```python
from build123d import *

# Parameters (mm, degrees)
SKETCH_R        = 4.3
SKETCH_R_2      = 2.8
PAD_DEPTH       = 10
SKETCH001_R     = 4.5
POCKET_DEPTH    = 5
FILLET_R        = 4
SKETCH002_R     = 4.3
POCKET001_DEPTH = 10.001


with BuildPart() as part:
    # Sketch → Pad (new body)
    with BuildSketch(Plane.XY):
        Polygon((0.4, 0), (177.6, 0), (177.6, 70), (115.6, 70), (115.6, 96.6), (-19, 96.6), (-19, 70.4), (0.4, 70.4), align=None)
        with Locations((15, 60)):
            Circle(SKETCH_R, mode=Mode.SUBTRACT)
        with Locations((15, 10)):
            Circle(SKETCH_R, mode=Mode.SUBTRACT)
        with Locations((170, 47)):
            Circle(SKETCH_R_2, mode=Mode.SUBTRACT)
        with Locations((170, 23)):
            Circle(SKETCH_R_2, mode=Mode.SUBTRACT)
    extrude(amount=PAD_DEPTH)

    # Sketch001 (on Face14 of Pad) → Pocket (cut)
    with BuildSketch(Plane.XY.offset(10)):
        with Locations((170, 47)):
            Circle(SKETCH001_R)
        with Locations((170, 23)):
            Circle(SKETCH001_R)
    extrude(amount=-POCKET_DEPTH, mode=Mode.SUBTRACT)

    # Fillet
    fillet_edges = [part.edges().sort_by_distance(p)[0] for p in [
        (115.6, 70, 5),
    ]]
    fillet(fillet_edges, radius=FILLET_R)

    # Sketch002 (on Face15 of Fillet) → Pocket001 (cut, through all)
    with BuildSketch(Plane.XY.offset(10)):
        with Locations((-11.5, 84.1)):
            Circle(SKETCH002_R)
        with Locations((23.5, 84.1)):
            Circle(SKETCH002_R)
        with Locations((103.1, 84.1)):
            Circle(SKETCH002_R)
    extrude(amount=-POCKET001_DEPTH, mode=Mode.SUBTRACT)


solid = part.part
```
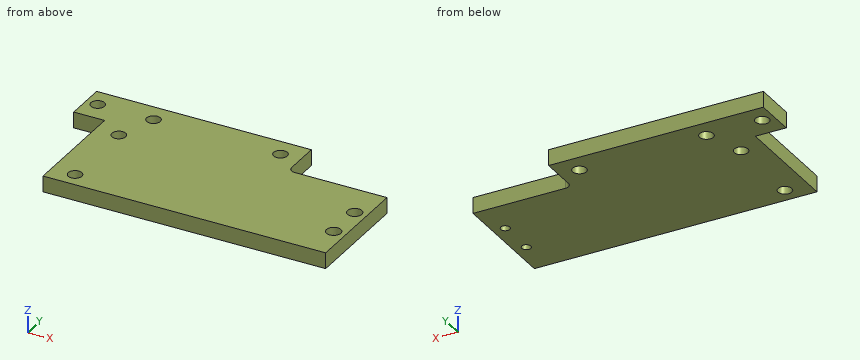
CAD build for the part. Positions are in the model's coordinates, mm. Give positions to 0.01 mm unless a question says otherwise; leave off trailing zeros. Loops run counter-clockwise (first coordinate to the right, second up) from the corner with the lowest first, then second, coordinate; pieces in that order, holes last. Notation, with made-up numbers: (-1, 57.5) - (4, 57.5) arc R19 cw to (4, 92.5) - close; hole circle Ø1 at (-29, 12.5). An arc over 180 degrees is marked (long way). Put each result on its own line as item: value.
Q1. Flat gauge pins, fed straight in: pin 1 (7 mm diameter, centred on x = 170, y = 23, fed in from +Z); pin 2 (5 mm diameter, centred on x = -8.5, z = 6.5, fed in from -Y); pin 3 (5 mm diameter, centred on y = 84, z = 5.5, fed in from +X); pin 4 (5 mm diameter, centred on x = 23.5, y = 84.1, fed in from -Z). Where does each tip first touch, or does it go through?
Filled in:
pin 1: stops at z = 5
pin 2: stops at y = 70.4
pin 3: stops at x = 115.6
pin 4: passes through
Q2. Slice it at B-B (y = 60). Give the cut face in (x, z), plus the area to 3 significant figures.
Filled in:
outline: (0.4, 0) - (10.7, 0) - (10.7, 10) - (0.4, 10) - close; (19.3, 0) - (177.6, 0) - (177.6, 10) - (19.3, 10) - close
area: 1,690 mm²
Q3. Slice it at A-A (y = 84.1). Give the cut face in (x, z).
Filled in:
outline: (-19, 0) - (-15.8, 0) - (-15.8, 10) - (-19, 10) - close; (-7.2, 0) - (19.2, 0) - (19.2, 10) - (-7.2, 10) - close; (27.8, 0) - (98.8, 0) - (98.8, 10) - (27.8, 10) - close; (107.4, 0) - (115.6, 0) - (115.6, 10) - (107.4, 10) - close
Q4. Probe line 1 along Y through (x, z) = (170, 3.45); line 2 along Y through (x, z) = (15, 2); line 3 along Y through (x, z) = (-11.5, 6). List the from-to ranges inside material, lowest first.
Filled in:
line 1: y = 0 to 20.2, 25.8 to 44.2, 49.8 to 70
line 2: y = 0 to 5.7, 14.3 to 55.7, 64.3 to 96.6
line 3: y = 70.4 to 79.8, 88.4 to 96.6
Q5. Slice it at C-C (x = 15). Give the cut face in (y, z).
Filled in:
outline: (0, 0) - (5.7, 0) - (5.7, 10) - (0, 10) - close; (14.3, 0) - (55.7, 0) - (55.7, 10) - (14.3, 10) - close; (64.3, 0) - (96.6, 0) - (96.6, 10) - (64.3, 10) - close
Q6. Slice it at D-D (z = 2.5). Give the cut face in (x, y), plus the area to 3 significant figures.
Filled in:
outline: (-19, 70.4) - (0.4, 70.4) - (0.4, 0) - (177.6, 0) - (177.6, 70) - (119.6, 70) arc R4 cw to (115.6, 74) - (115.6, 96.6) - (-19, 96.6) - close; hole circle Ø8.6 at (-11.5, 84.1); hole circle Ø8.6 at (15, 10); hole circle Ø8.6 at (15, 60); hole circle Ø8.6 at (23.5, 84.1); hole circle Ø8.6 at (103.1, 84.1); hole circle Ø5.6 at (170, 23); hole circle Ø5.6 at (170, 47)
area: 15,600 mm²
